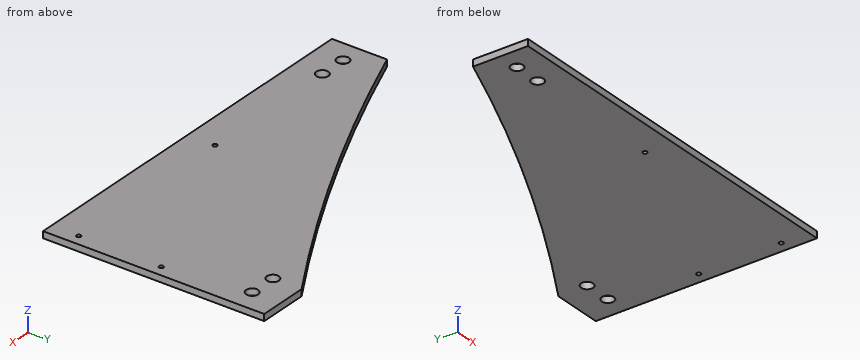
Autodesk Inventor part; units mm, degrees
ref_plane "YZ Plane" through (0, 0, 0) normal (1, 0, 0) x (0, 1, 0)
ref_plane "XZ Plane" through (0, 0, 0) normal (0, 1, 0) x (-1, 0, 0)
ref_plane "XY Plane" through (0, 0, 0) normal (0, 0, 1) x (1, 0, 0)
sketch "Sketch1" plane through (0, 0, 0) normal (0, 0, 1) x (1, 0, 0)
  line L0 (0, 0) -> (700, 0)
  line L1 (0, 0) -> (0, 100)
  circle A0 centre (40, 50) radius 10.95
  circle A1 centre (90, 50) radius 10.95
  circle A2 centre (609.6152, 350) radius 10.95
  circle A3 centre (659.6152, 350) radius 10.95
  line L2 (700, 0) -> (700, 402.1837)
  line L3 (700, 402.1837) -> (609.6152, 402.1837)
  arc A4 (0, 100) -> (609.6152, 402.1837) centre (-1371.2256, 3632.2653) ccw
  circle A5 centre (350, 50) radius 3.95
  circle A6 centre (680, 50) radius 3.95
  circle A7 centre (680, 200) radius 3.95
  dimension "d0" = 700
  dimension "d1" = 100
  dimension "d3" = 21.9
  dimension "d5" = 21.9
  dimension "d9" = 21.9
  dimension "d10" = 21.9
  dimension "d14" = 7.9
  dimension "d17" = 7.9
  dimension "d18" = 7.9
extrude "Plate1" add sketch "Sketch1" along normal blind 12
equation "\"d19\" = Thickness"
equation "\"BendRadius\" = Thickness"
equation "\"BendReliefWidth\" = Thickness"
equation "\"BendReliefDepth\" = 0.5 * Thickness"
equation "\"CornerReliefSize\" = 4 * Thickness"
equation "\"MinimumRemnant\" = 2 * Thickness"
equation "\"TransitionRadius\" = BendRadius"
equation "\"JacobiRadiusSize\" = BendRadius"
equation "\"GapSize\" = Thickness"
properties part number "Laser Print For Left Frame with support"
Build history of the part. All positions in model axes, mm. Give positions to 0.01 mm unless a question says otherwise; leave off trailing zeros. Order: outer loops, then holes, each group sorted by start corner. A loop starts at its lowest first (then second) coordinate and runs counter-clockwise, first axis right, second up. Notation, with made-up numbers: M 9.5,26 L 49.5,26 A14 cw 49.5,38 Z; hole C 68.25,7.5 d6. An arc over 180 degrees is marked long. Return JSON: item names as keys, results as strings.
Q1. Band-saw the part on A-A (y = 350). Give the cut face in (x, z).
Answer list:
{"outline": "M 521.89,0 L 598.67,0 L 598.67,12 L 521.89,12 Z; M 620.57,0 L 648.67,0 L 648.67,12 L 620.57,12 Z; M 670.57,0 L 700,0 L 700,12 L 670.57,12 Z"}
Q2. Flat gauge pins, fed straight in: pin 1 (5 mm diameter, centred on x = 448, z = 3.5, fed in from +Y); pin 2 (3 mm diameter, centred on x = 519, z = 4.5, fed in from +Y); pin 3 (10.5 mm diameter, centred on x = 350, y = 50, fed in from +Z); pin 4 (3 mm diameter, centred on x = 464.5, z = 10.5, fed in from +Y). Where does each tip first touch, or does it go through?
Answer list:
{"pin 1": "stops at y = 309.85", "pin 2": "stops at y = 349.2", "pin 3": "stops at z = 12", "pin 4": "stops at y = 318.39"}
Q3. Band-saw the part on D-D (y = 243.5). Give the cut face in (x, z), then the cut area to 3 significant figures.
Answer list:
{"outline": "M 323.89,0 L 700,0 L 700,12 L 323.89,12 Z", "area": "4,510 mm^2"}
Q4. Band-saw the part on B-B (z = 3.5). Give the cut face in (x, y), then the cut area to 3 significant figures.
Answer list:
{"outline": "M 0,0 L 700,0 L 700,402.18 L 609.62,402.18 A3789.08 cw 0,100 Z; hole C 40,50 d21.9; hole C 90,50 d21.9; hole C 350,50 d7.9; hole C 609.62,350 d21.9; hole C 659.62,350 d21.9; hole C 680,50 d7.9; hole C 680,200 d7.9", "area": "181,000 mm^2"}
Q5. Wall check: probe 1 along X at (y, z) = (349, 7.75); probe 2 along X at (y, z) = (342, 4.25); probe 3 along Y at (x, z) = (668.5, 3.5). Give the ranges that are in metal, low to high. Write a range as from..to.
Answer list:
{"probe 1": "x = 520.16..598.71, 620.52..648.71, 670.52..700", "probe 2": "x = 507.95..602.14, 617.09..652.14, 667.09..700", "probe 3": "y = 0..343.6, 356.4..402.18"}
Q6. Band-saw the part on C-C (x = 124). Give the cut face in (y, z).
Answer list:
{"outline": "M 0,0 L 150.68,0 L 150.68,12 L 0,12 Z"}
